Source: CAD feature listing. Evaluate the final solid. Frame: model axes, mm. A direction names the side the tool comes from. Coordinates: 2 decimals unless noted, no trailing zeros. Write each loop counter-clockwise with the first axis right and the second up, starting at its lowest first coordinate (ties: lowest second). Pieces come first, ordered by that corner, then holes. Notation, with made-up numbers: M -11,74.25 L 46,74.25 A26 cw 46,91.25 Z; hole C -11,-38.75 d1. An arc over 180 degrees is marked long. One line per item, written item: value. Start each with the question number.
Item 1: Set-up query: faces 1 (the flat face through (15, 101, 0)), 2 (the flat face through (0, 25, 0)). Return all of +Z, -Z, +X, -X, +Y, -Y with unobstructed straight access to the full face (end or side cutting, diameter ignored); none if empty.
Item 2: Cut plane B-B, the plane z = -7. Output: boundary loops of the cut face in (x, y), then the cut area to 3 significant figures.
Item 3: Cut plane A-A, the plane y = 63. Output: boundary loops of the cut face in (x, z).
Item 4: Pin query (flat end, axial travel): P1, Ø6, axis at x = -4, y = 95.5, coming from the +Z side; P2, Ø1.5, axis at x = -7.5, z = -1.5, coming from the -Y side. Return the tip coordinate at first contact, or that it passes through.
Item 5: Ray query, L1, parallel to Z at x = 0, y = 14.75; L2, parallel to Y at x = 7.25, z = 0; L3, parallel to Z at x = 12.25, y = 10. Return the intervals inside material, ascending. Write a range as from..to.
Item 6: Mould query, pull axis X, two halves, no side actions, for faces 3 (the cylindrical face through (-14.99, 98.6, -0.59)), 4 (the flat face through (0, 200, 0)), 5 (the cylindrical face through (-2, 12, 0)). Classes: released by +X, released by -X, zero draft, split by the parting line, or undercut.
```python
from build123d import *

# Parameters (mm, degrees)
SKETCH1_R           = 15
BOSS_EXTRUDE1_DEPTH = 200
SKETCH2_W           = 0.857864376
SKETCH2_H           = 10
BOSS_EXTRUDE2_DEPTH = 200
CUT_EXTRUDE1_DEPTH  = 25
SKETCH4_R           = 1.5
CUT_EXTRUDE2_DEPTH  = 15


with BuildPart() as part:
    # Sketch1 → Boss-Extrude1 (new body)
    with BuildSketch(Plane(origin=(0, 0, 0), x_dir=(1, 0, 0), z_dir=(0, 1, 0))):
        with Locations(Location((0, 0, 0), (0, 0, 270))):
            Circle(SKETCH1_R)
    extrude(amount=BOSS_EXTRUDE1_DEPTH)

    # Sketch2 → Boss-Extrude2 (add)
    with BuildSketch(Plane(origin=(0, 200, 0), x_dir=(1, 0, 0), z_dir=(0, 1, 0))):
        with Locations((14.571067812, 0)):
            Rectangle(SKETCH2_W, SKETCH2_H)
    extrude(amount=-BOSS_EXTRUDE2_DEPTH)

    # Sketch3 → Cut-Extrude1 (cut)
    with BuildSketch(Plane.XZ):
        with BuildLine():
            Line((1.5, -1.322875656), (1.5, 1.322875656))
            ThreePointArc((1.5, 1.322875656), (-2, 0), (1.5, -1.322875656))
        make_face()
    extrude(amount=-CUT_EXTRUDE1_DEPTH, mode=Mode.SUBTRACT)

    # Sketch4 → Cut-Extrude2 (cut)
    with BuildSketch(Plane(origin=(15, 0, 0), x_dir=(0, 0, -1), z_dir=(1, 0, 0))):
        with Locations((0, 10)):
            Circle(SKETCH4_R)
    extrude(amount=-CUT_EXTRUDE2_DEPTH, mode=Mode.SUBTRACT)


solid = part.part
```
From the geometry:
1. face 1: +Z, -Z, +X, +Y, -Y
1. face 2: -Y
2. outline: M -13.27,0 L 13.27,0 L 13.27,200 L -13.27,200 Z
2. area: 5,310 mm²
3. outline: M 14.14,-5 L 15,-5 L 15,5 L 14.14,5 A15 ccw long Z
4. P1: stops at z = 14.97
4. P2: stops at y = 0
5. L1: z = -15..-2, 2..15
5. L2: y = 0..8.5, 11.5..200
5. L3: z = -8.66..-1.5, 1.5..8.66
6. face 3: split by the parting line
6. face 4: zero draft
6. face 5: undercut
